The model under review builds one solid part; all positions refer to its coordinate system, in mm. A direction names the side the tool comes from. Give positions to 0.01 mm unless a question says otherwise; leave off trailing zeros. Order: outer loops, then holes, each group sorted by start corner. A loop starts at its lowest first (then second) coordinate and runs counter-clockwise, first axis right, second up.
```python
from build123d import *

# Parameters (mm, degrees)
F0_W     = 152.4
F0_H     = 101.6
F1_DEPTH = 76.2
F3_DEPTH = 152.654
F4_W     = 12.7030066214
F4_H     = 9.8352176327
F4_H_2   = 45.31371966
F5_DEPTH = 115.316
F6_R     = 22.86
F7_DEPTH = 193.04


with BuildPart() as f1:
    # F0 (on Top) → F1 (new body)
    with BuildSketch(Plane.XY):
        with Locations((34.5954637319, 4.3489372927)):
            Rectangle(F0_W, F0_H)
    extrude(amount=F1_DEPTH)

    # F2 (on face) → F3 (cut)
    with BuildSketch(Plane(origin=(-41.6045362681, 0, 0), x_dir=(0, -1, 0), z_dir=(-1, 0, 0))):
        with BuildLine():
            Line((34.8858758807, 76.2), (-45.31371966, 76.2))
            ThreePointArc((-45.31371966, 76.2), (-5.2139218897, 42.5794624331), (34.8858758807, 76.2))
        make_face()
    extrude(amount=-F3_DEPTH, mode=Mode.SUBTRACT)

    # F4 (on face) → F5 (cut)
    with BuildSketch(Plane.XY.offset(76.2)):
        with Locations((35.3598685469, 50.2313284764)):
            Rectangle(F4_W, F4_H)
        with Locations((35.3598685469, 22.65685983)):
            Rectangle(F4_W, F4_H_2)
    extrude(amount=-F5_DEPTH, mode=Mode.SUBTRACT)

    # F6 (on face) → F7 (cut)
    with BuildSketch(Plane(origin=(-41.6045362681, 0, 0), x_dir=(0, -1, 0), z_dir=(-1, 0, 0))):
        with Locations((21.8480825203, 24.0417348414)):
            Circle(F6_R)
    extrude(amount=-F7_DEPTH, mode=Mode.SUBTRACT)


solid = f1.part
```
Item 1: Take a section at D-D (x = 38). Give the boundary of the cut face in (y, z).
Values found:
outline: (-46.45, 0) - (0, 0) - (0, 17.32) arc R22.86 cw (long way) to (0, 30.77) - (0, 42.91) arc R40.72 cw to (-34.89, 76.2) - (-46.45, 76.2) - close
Item 2: Take a section at A-A (z = 29). Give the boundary of the cut face in (x, y).
Values found:
outline: (-41.6, -46.45) - (110.8, -46.45) - (110.8, -44.16) - (-41.6, -44.16) - close; (-41.6, 0.47) - (29.01, 0.47) - (29.01, 55.15) - (-41.6, 55.15) - close; (41.71, 0.47) - (110.8, 0.47) - (110.8, 55.15) - (41.71, 55.15) - close
Item 3: Take a section at C-C (z = 38). Give the boundary of the cut face in (x, y).
Values found:
outline: (-41.6, -46.45) - (110.8, -46.45) - (110.8, -39.95) - (-41.6, -39.95) - close; (-41.6, -3.74) - (110.8, -3.74) - (110.8, 55.15) - (41.71, 55.15) - (41.71, 0) - (29.01, 0) - (29.01, 55.15) - (-41.6, 55.15) - close
Item 4: Clearance check with flat-ended pins moving along their axes: pin 1 Ø5 at (x, y) = (38, 28) entering from +Z; pin 2 Ø10 at (x, y) = (-6.5, -8.5) entering from +Z; pin 3 Ø6 at (x, z) = (38.5, 38) entering from +Y. State where each tip first meets the part, or that it passes through.
Values found:
pin 1: passes through
pin 2: stops at z = 47.13
pin 3: stops at y = 0
Item 5: For faces 4 (the flat face through (35, 0, 9)), 5 (the flat face through (-7, 50, 76.2)), list the 3-axis set-ups (+Z, -Z, +X, -X, +Y, -Y) from which the entire face can be reached by the end or side of a thin tool; tool diameter is ignored.
Values found:
face 4: +Z, -Z, +Y
face 5: +Z, +X, -X, +Y, -Y
Item 6: For line 1 (X direction, y = 41, z = 45.5); line 2 (Y direction, x = -21, z = 31); line 3 (Y direction, x = -28, z = 15), list the stretches that pass through material, from the lowest coordinate up.
Values found:
line 1: x = -41.6 to 29.01, 41.71 to 110.8
line 2: y = -46.45 to -43.62, -0.07 to 55.15
line 3: y = -46.45 to -42.84, -0.85 to 55.15
Item 7: Take a section at B-B (y = -2). Give the boundary of the cut face in (x, z), and give its area (3 significant figures).
Values found:
outline: (-41.6, 0) - (110.8, 0) - (110.8, 12.7) - (-41.6, 12.7) - close; (-41.6, 35.38) - (110.8, 35.38) - (110.8, 43.22) - (-41.6, 43.22) - close
area: 3,130 mm2
Item 8: Draft analysis for pull direction X (two halves, no side actions). For faces 1 (the flat face through (34, -6, 0)), 2 (the flat face through (-41.605, 15, 29)), 3 (the flat face through (29.008, 34, 30)), state which applies: released by +X, released by -X, zero draft, split by the parting line, or undercut.
Values found:
face 1: zero draft
face 2: released by -X
face 3: undercut
